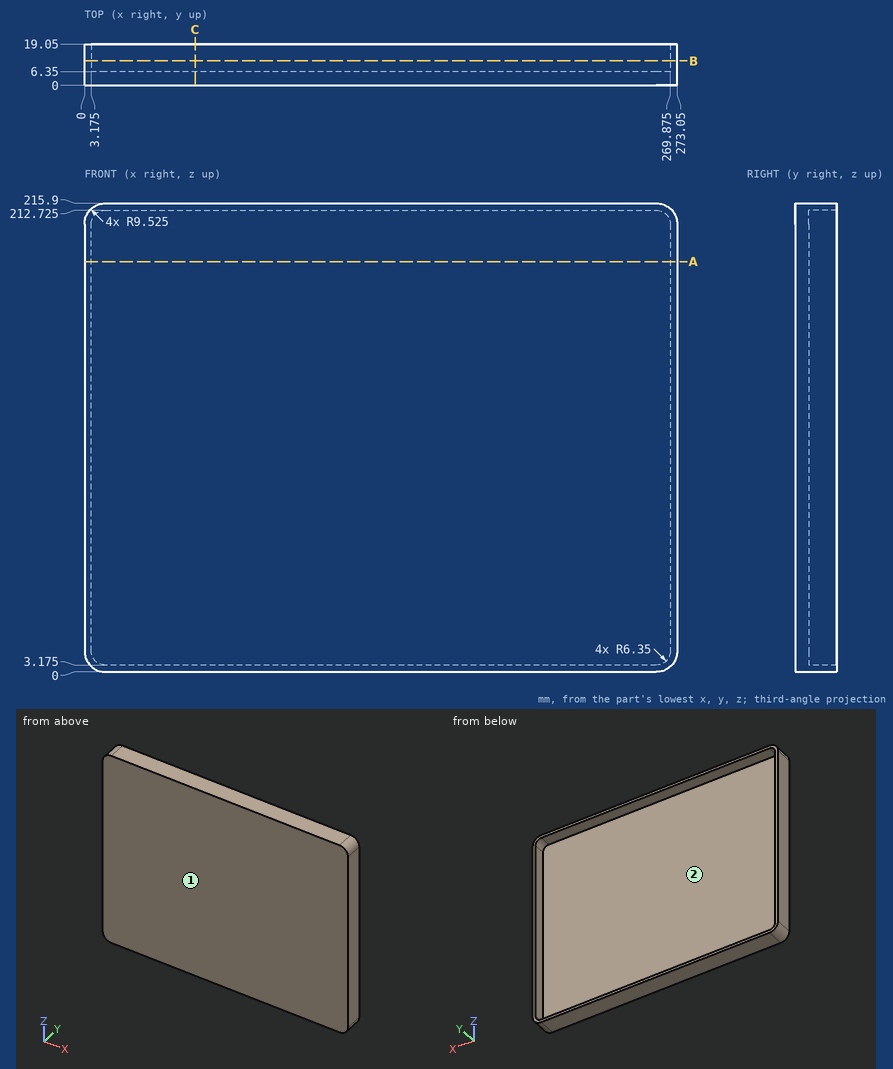
For this review, use the dimensioned drawing (mm, ordinates from the lowest corner) and the shaded views. Coordinates: 2 decimals unless noted, no trailing zeros. Write each loop counter-clockwise with the first axis right and the second up, starting at its lowest first coordinate (ties: lowest second). Pieces come first, ordered by that corner, then holes. Notation, with made-up numbers: (-12, 49) - (14, 49) arc R20 cw to (14, 77) - close; hole circle Ø10 at (85.25, 84.25). An arc over 180 degrees is marked (long way). Answer in a Markdown table with one row per item. Add a question column.
Q1. Consider section C-C on x = 51. Give the boundary of the cut face in (y, z) (3 decimals).
Q2. Consider section A-A on z = 189. Give the boundary of the cut face in (x, y) (3 decimals).
Q3. To check wall thickness, follow line 1 along Z through (x, y) = (80, 7) (3 decimals); line 2 along X through (y, z) = (9.5, 176) (3 decimals); line 3 along Y through (x, z) = (148.5, 26.5). State the ranges of each line that lie inside material, in increasing order. Write a range as from..to.
Q4. Draft analysis for pull direction X (two halves, no side actions). For the marked faces 1 and 2, state which applies: +X half, -X half, draft (parallel to the pull), parting line (faces both ways), or undercut.
Q5. Consider section B-B on y = 11.25. Give the boundary of the cut face in (x, z) (3 decimals), then the cut area to 3 significant figures.
Answers below:
| question | item | result |
|---|---|---|
| 1 | outline | (0, 0) - (19.05, 0) - (19.05, 3.175) - (6.35, 3.175) - (6.35, 212.725) - (19.05, 212.725) - (19.05, 215.9) - (0, 215.9) - close |
| 2 | outline | (0, 0) - (273.05, 0) - (273.05, 19.05) - (269.875, 19.05) - (269.875, 6.35) - (3.175, 6.35) - (3.175, 19.05) - (0, 19.05) - close |
| 3 | line 1 | 0..3.175, 212.725..215.9 |
| 3 | line 2 | 0..3.175, 269.875..273.05 |
| 3 | line 3 | 0..6.35 |
| 4 | face 1 | draft |
| 4 | face 2 | undercut |
| 5 | outline | (0, 9.525) arc R9.525 ccw to (9.525, 0) - (263.525, 0) arc R9.525 ccw to (273.05, 9.525) - (273.05, 206.375) arc R9.525 ccw to (263.525, 215.9) - (9.525, 215.9) arc R9.525 ccw to (0, 206.375) - close; hole (3.175, 9.525) arc R6.35 ccw to (9.525, 3.175) - (263.525, 3.175) arc R6.35 ccw to (269.875, 9.525) - (269.875, 206.375) arc R6.35 ccw to (263.525, 212.725) - (9.525, 212.725) arc R6.35 ccw to (3.175, 206.375) - close |
| 5 | area | 3,020 mm² |
